from build123d import *

# Parameters (mm, degrees)
SCHIZZO1_R                   = 6.25
ESTRUSIONE_ESTRUSIONE1_DEPTH = 6


with BuildPart() as part:
    # Schizzo1 → Estrusione-Estrusione1 (new body)
    with BuildSketch(Plane.XY):
        with BuildLine():
            Line((0, 0), (-19.5, 0))
            Line((-19.5, 0), (-19.5, -10))
            ThreePointArc((-19.5, -10), (-23.5, -14), (-27.5, -10))
            Line((-27.5, -10), (-27.5, 15))
            Line((-27.5, 15), (8.032195982, 15))
            Line((8.032195982, 15), (20, 15))
            ThreePointArc((20, 15), (42.5, 7.5), (20, 0))
            Line((20, 0), (0, 0))
        make_face()
        with Locations((0, 7.5)):
            Circle(SCHIZZO1_R, mode=Mode.SUBTRACT)
    extrude(amount=ESTRUSIONE_ESTRUSIONE1_DEPTH)


solid = part.part
Design review of the part built by this model. Coordinates are the model's own, in mm. A direction names the side the tool comes from. Round coordinates to 2 decimals unless told otherwise and drop trailing zeros. Loops run counter-clockwise (first coordinate to the right, second up) from the corner with the lowest first, then second, coordinate; pieces in that order, holes last. Notation, with made-up numbers: (49, -19) - (67, -19) arc R25 cw to (67, 20) - close; hole circle Ø5 at (28.5, 38). An arc over 180 degrees is marked (long way). One line per item, written item: value. Start each with the question number.
1) Insertion check: pin 1 Ø1 at (x, z) = (-4.5, 4.5) entering from +Y; pin 2 Ø2 at (y, z) = (12.5, 3.5) entering from +X; pin 3 Ø1 at (y, z) = (5.5, 1.5) entering from +X; pin 4 Ø7.5 at (x, y) = (0, 7.5) entering from -Z. Each pin has a flat end and moves straight along its axis. Give the tip position at first contact, or say it passes through.
2) Consider section C-C on y = 10. Give the boundary of the cut face in (x, z), then the cut area to 3 significant figures.
3) Consider section A-A on x = 0. Give the boundary of the cut face in (y, z), then the cut area to 3 significant figures.
4) To check wall thickness, follow L1, parallel to Y at x = 0, z = 2.6; L2, parallel to Y at x = -9, z = 0.8; L3, parallel to Y at x = -5, z = 1.6. State the ranges of each line that lie inside material, in increasing order. Write a range as from..to.
5) Draft analysis for pull direction Y (two halves, no side actions). For faces 1 (the flat face through (-27.5, 2, 3)), 2 (the cylindrical face through (2.884, 1.955, 2.958)), 3 (the cylindrical face through (-23.4, -14, 3)), state which applies: +Y half, -Y half, draft (parallel to the pull), parting line (faces both ways), or undercut.
6) Consider section D-D on x = 30. Give the boundary of the cut face in (y, z).
7) Consider section B-B on z = 1.65. Give the boundary of the cut face in (x, y), then the cut area to 3 significant figures.
8) For faces 4 (the flat face through (1, 0, 3)), 5 (the flat face through (-4, 15, 3)), 6 (the flat face through (8, 7, 0)), list the 3-axis set-ups (+Z, -Z, +X, -X, +Y, -Y) from which the entire face can be reached by the end or side of a thin tool; tool diameter is ignored.
Reported:
1. pin 1: stops at y = 15
1. pin 2: stops at x = 41.84
1. pin 3: stops at x = 42.41
1. pin 4: passes through
2. outline: (-27.5, 0) - (-5.73, 0) - (-5.73, 6) - (-27.5, 6) - close; (5.73, 0) - (42.25, 0) - (42.25, 6) - (5.73, 6) - close
2. area: 350 mm^2
3. outline: (0, 0) - (1.25, 0) - (1.25, 6) - (0, 6) - close; (13.75, 0) - (15, 0) - (15, 6) - (13.75, 6) - close
3. area: 15.0 mm^2
4. L1: y = 0..1.25, 13.75..15
4. L2: y = 0..15
4. L3: y = 0..3.75, 11.25..15
5. face 1: draft
5. face 2: undercut
5. face 3: -Y half
6. outline: (-5, 0) - (20, 0) - (20, 6) - (-5, 6) - close
7. outline: (-27.5, -10) arc R4 ccw to (-19.5, -10) - (-19.5, 0) - (20, 0) arc R12.5 ccw (long way) to (20, 15) - (-27.5, 15) - close; hole circle Ø12.5 at (0, 7.5)
7. area: 1,160 mm^2
8. face 4: +Z, -Z, -Y
8. face 5: +Z, -Z, -X, +Y
8. face 6: -Z, +X, -X, +Y, -Y
